Build history of the part. All positions in model axes, mm. Coordinates: 2 decimals unless noted, no trailing zeros. Order: outer loops, then holes, each group sorted by start corner. A loop starts at its lowest first (then second) coordinate and runs counter-clockwise, first axis right, second up. Notation, with made-up numbers: (-18.5, -25) -> (-3.5, -25) arc R19 cw to (-3.5, -2) -> close; hole circle Ø5 at (31.5, 59.5). An arc over 180 degrees is marked (long way). Write each question's results on one line, items separated by ' | '.
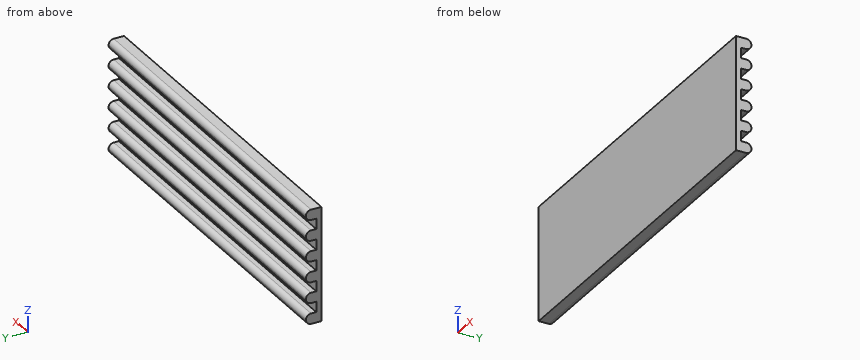
from build123d import *

# Parameters (mm, degrees)
SKETCH_1_W          = 70
SKETCH_1_H          = 22
EXTRUDE_1_DEPTH     = 3
SKETCH_2_W          = 35
SKETCH_2_H          = 2
CUT_EXTRUDE_1_DEPTH = 2
FILLET_1_R          = 1


with BuildPart() as part:
    # 草图1 → 凸台-拉伸1 (new body)
    with BuildSketch(Plane(origin=(0, 0, 0), x_dir=(1, 0, 0), z_dir=(0, 1, 0))):
        Rectangle(SKETCH_1_W, SKETCH_1_H)
    extrude(amount=EXTRUDE_1_DEPTH)

    # 草图2 → 切除-拉伸1 (cut)
    with BuildSketch(Plane(origin=(0, 3, 0), x_dir=(1, 0, 0), z_dir=(0, 1, 0))):
        with Locations((17.5, -8)):
            Rectangle(SKETCH_2_W, SKETCH_2_H)
        with Locations((-17.5, -8)):
            Rectangle(SKETCH_2_W, SKETCH_2_H)
        with Locations((-17.5, -4)):
            Rectangle(SKETCH_2_W, SKETCH_2_H)
        with Locations((17.5, -4)):
            Rectangle(SKETCH_2_W, SKETCH_2_H)
        with Locations((17.5, 0)):
            Rectangle(SKETCH_2_W, SKETCH_2_H)
        with Locations((-17.5, 0)):
            Rectangle(SKETCH_2_W, SKETCH_2_H)
        with Locations((-17.5, 4)):
            Rectangle(SKETCH_2_W, SKETCH_2_H)
        with Locations((17.5, 4)):
            Rectangle(SKETCH_2_W, SKETCH_2_H)
        with Locations((17.5, 8)):
            Rectangle(SKETCH_2_W, SKETCH_2_H)
        with Locations((-17.5, 8)):
            Rectangle(SKETCH_2_W, SKETCH_2_H)
    extrude(amount=-CUT_EXTRUDE_1_DEPTH, mode=Mode.SUBTRACT)

    # 圆角1
    fillet_1_edges = [part.edges().sort_by_distance(p)[0] for p in [
        (0, 3, 11),
        (0, 3, 9),
        (0, 3, 7),
        (0, 3, 5),
        (0, 3, 3),
        (0, 3, 1),
        (0, 3, -1),
        (0, 3, -3),
        (0, 3, -5),
        (0, 3, -7),
        (0, 3, -9),
        (0, 3, -11),
    ]]
    fillet(fillet_1_edges, radius=FILLET_1_R - 0.0001)  # a hair under: the kernel refuses the full size


solid = part.part
Item 1: Slice it at A-A, the plane y = 2.55. List the corners of the cut face in (x, z), and give its area (3 significant figures).
Answer:
outline: (-35, -10.84) -> (35, -10.84) -> (35, -9.16) -> (-35, -9.16) -> close; (-35, -6.84) -> (35, -6.84) -> (35, -5.16) -> (-35, -5.16) -> close; (-35, -2.84) -> (35, -2.84) -> (35, -1.16) -> (-35, -1.16) -> close; (-35, 1.16) -> (35, 1.16) -> (35, 2.84) -> (-35, 2.84) -> close; (-35, 5.16) -> (35, 5.16) -> (35, 6.84) -> (-35, 6.84) -> close; (-35, 9.16) -> (35, 9.16) -> (35, 10.84) -> (-35, 10.84) -> close | area: 702 mm^2
Item 2: Drill centre lines: line 1 (Z direction, x = 1.5, y = 1.4); line 2 (Z direction, x = 21.5, y = 2.35); line 3 (Y direction, x = 11.5, z = -4.5). Where is each one in solid material? Low to high. Write a range as from..to.
Answer:
line 1: z = -11..-9, -7..-5, -3..-1, 1..3, 5..7, 9..11 | line 2: z = -10.94..-9.06, -6.94..-5.06, -2.94..-1.06, 1.06..2.94, 5.06..6.94, 9.06..10.94 | line 3: y = 0..1
Item 3: Pin check, flat tips, straight feed: pin 1 (1 mm diameter, centred on x = 20, z = -3, fed in from +Y); pin 2 (1 mm diameter, centred on x = 12.5, z = -8, fed in from +Y); pin 3 (1.6 mm diameter, centred on x = -4, z = 4.5, fed in from +Y). Stop position of each tip, or through.
Answer:
pin 1: stops at y = 2.87 | pin 2: stops at y = 1 | pin 3: stops at y = 2.71
